Input: part model. Units: mm. Frame: model coordinates. A direction names the side the tool comes from. Round coordinates to 2 decimals unless told otherwise and drop trailing zeros. Loops run counter-clockwise (first coordinate to the right, second up) from the corner with the lowest first, then second, coordinate; pieces in that order, holes last.
1) Access query for faces 1 (the face through (0, 20, -31)), 2 (the face through (14.625, 5, -53)). Directions: +Z, -Z, +X, -X, +Y, -Y. A direction counts if a zero-diameter tool reaches every point of the face in a straight line with its end or side. Return the directions, or none.
2) Draft query along Z for faces 3 (the face through (0, 5, -77.5)), 4 (the face through (-19.894, 5, -31)), 5 (the face through (-9.375, 5, -10)). Return one class per face: pulls with the +Z half, pulls with the -Z half, needs draft (parallel to the pull), parting line crosses it, or undercut.
3) Section B-B, the plane z = -56. Return loops of the section in (x, y) (3 decimals).
4) Section A-A, the plane x = 0. Return loops of the section in (y, z), and give its area (3 significant figures).
5) Section C-C, the plane z = -31.5. Return loops of the section in (x, y), and give its area (3 significant figures).
6) Ray query, line 1 along X through (y, z) = (6.75, 2) (3 decimals); line 2 along X through (y, z) = (9.5, -48.5) (3 decimals); line 3 along Z through (x, y) = (-2.5, 7.25). Return the intervals inside material, ascending.
7) First-contact query: pin 1 (20 mm diameter, centred on x = 9.5, z = -50.5, fed in from +Y); pin 2 (1.5 mm diameter, centred on x = -1.5, y = 15, fed in from +Z). Flat tips, straight axial feed; report the tip coordinate or a pass-through.
8) Section D-D, the plane y = 8. State how many separate pieces and enclosed holes the cut face has, and give its area (3 significant figures).
from build123d import *

# Parameters (mm, degrees)
BOSS_EXTRUDE1_DEPTH  = 10
FILLET2_R            = 1
FILLET2_OF_MIRROR1_R = 1
CUT_EXTRUDE1_DEPTH   = 81.635062113
FILLET3_R            = 1
SKETCH5_R            = 2.5
BOSS_EXTRUDE2_DEPTH  = 10
FILLET1_R            = 0.5


with BuildPart() as part:
    # Sketch2 → Boss-Extrude1 (new body)
    with BuildSketch(Plane(origin=(0, 0, 0), x_dir=(1, 0, 0), z_dir=(0, 1, 0))):
        Polygon((-19.893799085, 77.5), (0, 77.5), (0, 75.5), (-2.625, 75.5), (-2.625, 73), (-2.625, 63), (-2.625, 60.5), (0, 60.5), (0, 60.375), (0, 2.5), (-2.625, 2.5), (-2.625, 0), (-2.625, -10), (-2.625, -12.5), (0, -12.5), (0, -14.5), (-19.893799085, -14.5), align=None)
    boss_extrude1 = extrude(amount=BOSS_EXTRUDE1_DEPTH)

    # Fillet2
    fillet2_edges = [part.edges().sort_by_distance(p)[0] for p in [
        (-2.625, 5, 12.5),
        (-2.625, 5, -2.5),
        (-2.625, 5, -60.5),
        (-2.625, 5, -75.5),
    ]]
    fillet(fillet2_edges, radius=FILLET2_R)

    # Mirror1: Boss-Extrude1 across Right Plane
    add(boss_extrude1.mirror(Plane(origin=(0, 0, 0), x_dir=(0, 0, -1), z_dir=(1, 0, 0))))

    # Fillet2 of Mirror1
    fillet2_of_mirror1_edges = [part.edges().sort_by_distance(p)[0] for p in [
        (2.625, 5, 12.5),
        (2.625, 5, -2.5),
        (2.625, 5, -60.5),
        (2.625, 5, -75.5),
    ]]
    fillet(fillet2_of_mirror1_edges, radius=FILLET2_OF_MIRROR1_R)

    # Sketch4 → Cut-Extrude1 (cut, through all)
    with BuildSketch(Plane(origin=(0, 0, 0), x_dir=(1, 0, 0), z_dir=(0, 1, 0))):
        Polygon((-14.625, 15), (-14.625, 5), (-14.625, 2.5), (-12, 2.5), (-9.375, 2.5), (-9.375, 5), (-9.375, 15), (-9.375, 17.5), (-12, 17.5), (-14.625, 17.5), align=None)
        Polygon((9.375, 58), (9.375, 48), (9.375, 45.5), (12, 45.5), (14.625, 45.5), (14.625, 48), (14.625, 58), (14.625, 60.5), (12, 60.5), (9.375, 60.5), align=None)
    extrude(amount=CUT_EXTRUDE1_DEPTH, mode=Mode.SUBTRACT)

    # Fillet3
    fillet3_edges = [part.edges().sort_by_distance(p)[0] for p in [
        (-14.625, 5, -17.5),
        (-14.625, 5, -2.5),
        (-9.375, 5, -2.5),
        (-9.375, 5, -17.5),
        (14.625, 5, -60.5),
        (9.375, 5, -60.5),
        (9.375, 5, -45.5),
        (14.625, 5, -45.5),
    ]]
    fillet(fillet3_edges, radius=FILLET3_R)

    # Sketch5 → Boss-Extrude2 (add)
    with BuildSketch(Plane(origin=(0, 10, 0), x_dir=(1, 0, 0), z_dir=(0, 1, 0))):
        with Locations(Location((0, 31.5, 0), (0, 0, 90))):
            Circle(SKETCH5_R)
    extrude(amount=BOSS_EXTRUDE2_DEPTH)

    # Fillet1
    fillet1_edges = [part.edges().sort_by_distance(p)[0] for p in [
        (0, 10, -29),
    ]]
    fillet(fillet1_edges, radius=FILLET1_R)


solid = part.part
Final values:
1. face 1: +Z, -Z, +X, -X, +Y
1. face 2: +Y, -Y
2. face 3: pulls with the -Z half
2. face 4: needs draft
2. face 5: undercut
3. outline: (-19.894, 0) - (9.375, 0) - (9.375, 10) - (-19.894, 10) - close; (14.625, 0) - (19.894, 0) - (19.894, 10) - (14.625, 10) - close
4. outline: (0, -77.5) - (10, -77.5) - (10, -75.5) - (0, -75.5) - close; (0, -60.5) - (10, -60.5) - (10, -34.5) arc R0.5 cw to (10.5, -34) - (20, -34) - (20, -29) - (10.5, -29) arc R0.5 cw to (10, -28.5) - (10, -2.5) - (0, -2.5) - close; (0, 12.5) - (10, 12.5) - (10, 14.5) - (0, 14.5) - close
4. area: 670 mm2
5. outline: (-19.89, 0) - (19.89, 0) - (19.89, 10) - (3, 10) arc R0.5 cw to (2.5, 10.5) - (2.5, 20) - (-2.5, 20) - (-2.5, 10.5) arc R0.5 cw to (-3, 10) - (-19.89, 10) - close
5. area: 448 mm2
6. line 1: x = -19.894 to -2.625, 2.625 to 19.894
6. line 2: x = -19.894 to 9.375, 14.625 to 19.894
6. line 3: z = -77.5 to -74.98, -61.02 to -1.98, 11.98 to 14.5
7. pin 1: stops at y = 10
7. pin 2: stops at z = -29.12
8. separate pieces: 1
8. enclosed holes: 4
8. area: 3,350 mm2
